```python
from build123d import *

# Parameters (mm, degrees)
SKETCH1_R           = 115
BOSS_EXTRUDE1_DEPTH = 30


with BuildPart() as part:
    # Sketch1 → Boss-Extrude1 (new body)
    with BuildSketch(Plane(origin=(0, 0, 0), x_dir=(1, 0, 0), z_dir=(0, 1, 0))):
        Circle(SKETCH1_R)
        with BuildLine():
            ThreePointArc((-3.955044182, 103.424405367), (-1.246353574, 103.492495393), (1.463191222, 103.489656833))
            Line((1.463191222, 103.489656833), (1.548013902, 109.489057229))
            ThreePointArc((1.548013902, 109.489057229), (40.682564415, 101.662082177), (74.412877774, 80.330402846))
            Line((74.412877774, 80.330402846), (70.335459814, 75.928736936))
            ThreePointArc((70.335459814, 75.928736936), (72.29894023, 74.061550359), (74.212870565, 72.143605694))
            Line((74.212870565, 72.143605694), (78.51506596, 76.325843705))
            ThreePointArc((78.51506596, 76.325843705), (100.652864871, 43.119030523), (109.420023069, 4.184322106))
            Line((109.420023069, 4.184322106), (103.424405367, 3.955044182))
            ThreePointArc((103.424405367, 3.955044182), (103.481099616, 1.977883277), (103.5, 0))
            ThreePointArc((103.5, 0), (103.497414176, -0.73161389), (103.489656833, -1.463191222))
            Line((103.489656833, -1.463191222), (109.489057229, -1.548013902))
            ThreePointArc((109.489057229, -1.548013902), (101.662082177, -40.682564415), (80.330402846, -74.412877774))
            Line((80.330402846, -74.412877774), (75.928736936, -70.335459814))
            ThreePointArc((75.928736936, -70.335459814), (74.061550359, -72.29894023), (72.143605694, -74.212870565))
            Line((72.143605694, -74.212870565), (76.325843705, -78.51506596))
            ThreePointArc((76.325843705, -78.51506596), (43.119030523, -100.652864871), (4.184322106, -109.420023069))
            Line((4.184322106, -109.420023069), (3.955044182, -103.424405367))
            ThreePointArc((3.955044182, -103.424405367), (1.246353574, -103.492495393), (-1.463191222, -103.489656833))
            Line((-1.463191222, -103.489656833), (-1.548013902, -109.489057229))
            ThreePointArc((-1.548013902, -109.489057229), (-40.682564415, -101.662082177), (-74.412877774, -80.330402846))
            Line((-74.412877774, -80.330402846), (-70.335459814, -75.928736936))
            ThreePointArc((-70.335459814, -75.928736936), (-72.29894023, -74.061550359), (-74.212870565, -72.143605694))
            Line((-74.212870565, -72.143605694), (-78.51506596, -76.325843705))
            ThreePointArc((-78.51506596, -76.325843705), (-100.652864871, -43.119030523), (-109.420023069, -4.184322106))
            Line((-109.420023069, -4.184322106), (-103.424405367, -3.955044182))
            ThreePointArc((-103.424405367, -3.955044182), (-103.492495393, -1.246353574), (-103.489656833, 1.463191222))
            Line((-103.489656833, 1.463191222), (-109.489057229, 1.548013902))
            ThreePointArc((-109.489057229, 1.548013902), (-101.662082177, 40.682564415), (-80.330402846, 74.412877774))
            Line((-80.330402846, 74.412877774), (-75.928736936, 70.335459814))
            ThreePointArc((-75.928736936, 70.335459814), (-74.061550359, 72.29894023), (-72.143605694, 74.212870565))
            Line((-72.143605694, 74.212870565), (-76.325843705, 78.51506596))
            ThreePointArc((-76.325843705, 78.51506596), (-43.119030523, 100.652864871), (-4.184322106, 109.420023069))
            Line((-4.184322106, 109.420023069), (-3.955044182, 103.424405367))
        make_face(mode=Mode.SUBTRACT)
    extrude(amount=BOSS_EXTRUDE1_DEPTH)


solid = part.part
```
Geometry check sheet. Reference: the model listing, model coordinates, mm. A direction names the side the tool comes from. Round coordinates to 2 decimals unless told otherwise and drop trailing zeros. Order: outer loops, then holes, each group sorted by start corner. A loop starts at its lowest first (then second) coordinate and runs counter-clockwise, first axis right, second up. Notation, with made-up numbers: (39.25, 83) - (64.25, 83) arc R13 cw to (64.25, 88) - close; hole circle Ø4 at (23.25, 8). An arc over 180 degrees is marked (long way). Use a Markdown table: item, result. Add a question column.
(1) Depth check by flat-ended pin: pin 1 (10 mm diameter, centred on x = 37.5, y = 25.5, fed in from -Z); pin 2 (10 mm diameter, centred on y = 13, z = -67, fed in from +X); pin 3 (1.5 mm diameter, centred on x = -10, y = 10, fed in from -Z); pin 4 (12 mm diameter, centred on x = -67, z = -81, fed in from -Y). Enter the tip coordinate at first touch or a pass-through.
(2) Sectioned sample at B-B, the plane x = 49. Enter the section's corners in (y, z), and give its area (3 significant figures).
(3) Material ranges on line 1 along X through (y, z) = (11.5, -71.5); line 2 along Z through (x, y) = (-76, 25); line 3 along X through (y, z) = (18, 72), recorded low to high. Write a range as [from, to].
(4) Release check for a two-part mould opening along Z. For faces 1 (the flat face through (106.46, 14.79, -4.07)), 2 (the flat face through (76, 30, 76)) record: pulls with the +Z half, pulls with the -Z half, needs draft (parallel to the pull), parting line crosses it, or undercut.
(5) Tool access check on faces 3 (the cylindrical face through (1.284, 14.79, 103.492)), 4 (the flat face through (76, 0, 76)). Record the directions out of +Z, -Z, +X, -X, +Y, -Y that give a thin tool (end or side, any length) a straight path to the whole face; none if there is none.
(6) Sectioned sample at A-A, the plane z = -47. Enter the section's corners in (x, y).
Answers below:
| question | item | result |
|---|---|---|
| 1 | pin 1 | z = -110.31 |
| 1 | pin 2 | x = 96.86 |
| 1 | pin 3 | z = -114.63 |
| 1 | pin 4 | y = 0 |
| 2 | outline | (0, -104.04) - (30, -104.04) - (30, -97.92) - (0, -97.92) - close; (0, 97.92) - (30, 97.92) - (30, 104.04) - (0, 104.04) - close |
| 2 | area | 367 mm² |
| 3 | line 1 | [-90.07, -82.93], [-77.19, -74.83], [82.93, 90.07] |
| 3 | line 2 | [-86.31, -78.83], [-78.18, -70.4], [73.88, 86.31] |
| 3 | line 3 | [-89.67, -82.5], [74.35, 77.73], [82.5, 89.67] |
| 4 | face 1 | undercut |
| 4 | face 2 | needs draft |
| 5 | face 3 | +Y, -Y |
| 5 | face 4 | +Z, -Z, +X, -X, -Y |
| 6 | outline | (-104.96, 0) - (-98.9, 0) - (-98.9, 30) - (-104.96, 30) - close; (98.9, 0) - (104.96, 0) - (104.96, 30) - (98.9, 30) - close |
